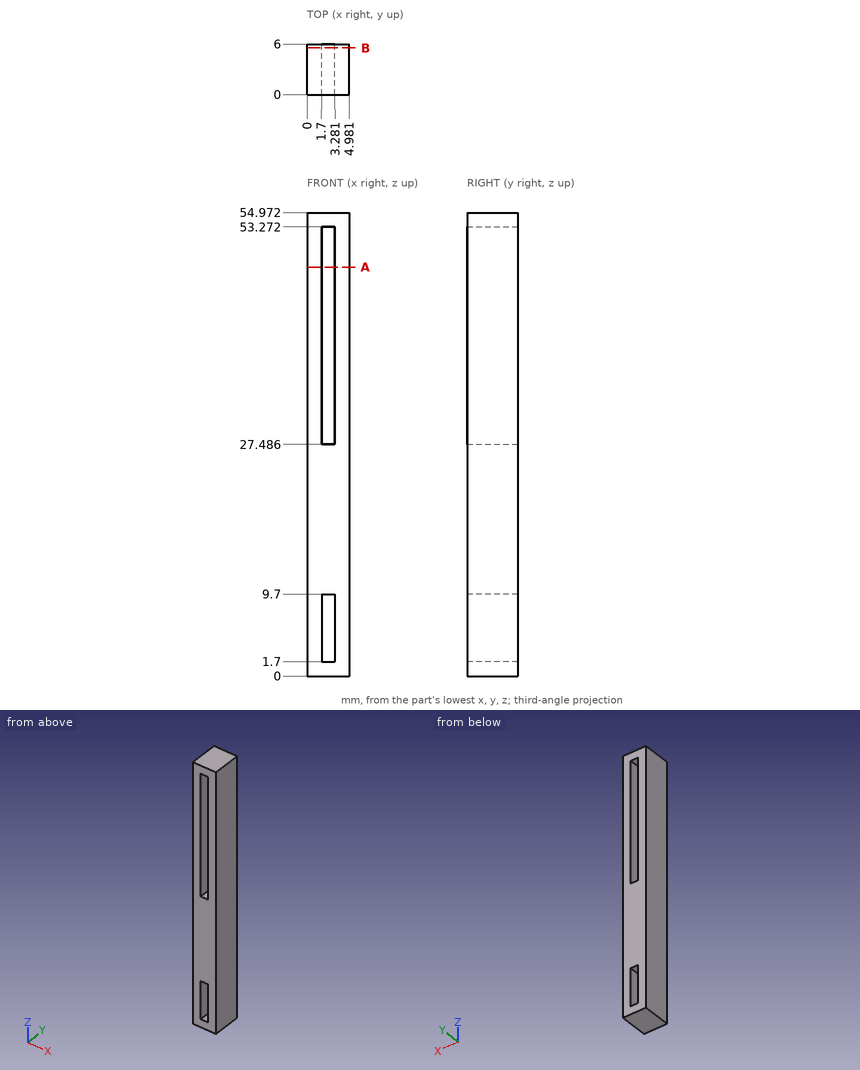
Design review of the part shown in the three views and the two pictorial views. Dimensions are in mm from the part's minimum x, y and z. Give positions to 0.01 mm unless a question says otherwise; leave off trailing zeros. Loops run counter-clockwise (first coordinate to the right, second up) from the corner with the lowest first, then second, coordinate; pieces in that order, holes last. Notation, with made-up numbers: M -12,61.25 L 27,61.25 A35 ccw 27,95.25 Z; hole C -2.75,62 d4. An arc over 180 degrees is marked long. Put each result on its own line as item: value. Start each with the question number.
(1) Add section A-A, the plane z = 48.5. Write out the cut boundary in (x, y), then the cut area to 3 significant figures.
(2) For pin 1 (1.5 mm diameter, centred on x = 3, z = 28.5, fed in from +Y), flat-tipped, find the tip position at first contact; note if it passes through.
(3) Add section B-B, the plane y = 5.55. Write out the cut boundary in (x, z).
(4) Wall thickness on L1, parallel to Z at x = 2.15, y = 4.05; L2, parallel to X at y = 2.7, z = 36.5: over which ranges is each line inside the solid? List them lowest first.
Result:
1. outline: M 0,0 L 1.7,0 L 1.7,6 L 0,6 Z; M 3.28,0 L 4.98,0 L 4.98,6 L 3.28,6 Z
1. area: 20.4 mm^2
2. pin 1: stops at y = 6
3. outline: M 0,0 L 4.98,0 L 4.98,54.97 L 0,54.97 Z; hole M 1.7,1.7 L 3.28,1.7 L 3.28,9.7 L 1.7,9.7 Z; hole M 1.7,27.49 L 3.28,27.49 L 3.28,53.27 L 1.7,53.27 Z
4. L1: z = 0 to 1.7, 9.7 to 27.49, 53.27 to 54.97
4. L2: x = 0 to 1.7, 3.28 to 4.98
